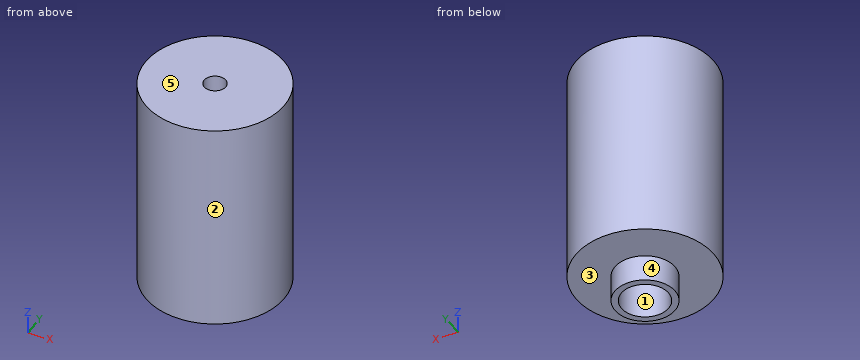
from build123d import *

# Parameters (mm, degrees)
SKETCH001_R   = 4.4
SKETCH001_R_2 = 2
PAD_DEPTH     = 4


with BuildPart() as part:
    # Sketch → Revolution (revolve)
    with BuildSketch(Plane.XZ):
        Polygon((-4.4, 0), (-5.6, 0), (-5.6, 5), (-12.85, 5), (-12.85, 45), (-4.4, 45), align=None)
    revolve(axis=Axis((0, 0, 0), (0, 0, 1)))

    # Sketch001 (on Face5 of Revolution) → Pad (new body)
    with BuildSketch(Plane(origin=(0, 0, 45), x_dir=(-1, 0, 0), z_dir=(0, 0, 1))):
        Circle(SKETCH001_R)
        Circle(SKETCH001_R_2, mode=Mode.SUBTRACT)
    extrude(amount=-PAD_DEPTH)


solid = part.part
Could you check a few things on this model? Use its own coordinates, in mm. Face numbers are marked on the shaded views. A direction names the side the tool comes from. Round coordinates to 2 decimals unless told otherwise and drop trailing zeros. Write each loop counter-clockwise with the first axis right and the second up, starting at its lowest first coordinate (ties: lowest second). Pieces come first, ordered by that corner, then holes. Notation, with made-up numbers: (4, 33) - (50, 33) arc R16 cw to (50, 50) - close; hole circle Ø3 at (22, -29.75). An arc over 180 degrees is marked (long way). Use a Markdown table: item, result.
Q1. Please list where these lines run through material, in increasing order: L1, parallel to Y at x = 0, z = 43.8; L2, parallel to Y at x = 0, z = 23.
Output values:
| item | result |
|---|---|
| L1 | -12.85 to -2, 2 to 12.85 |
| L2 | -12.85 to -4.4, 4.4 to 12.85 |
Q2. Thinking about a two-plate mould opening in Y: for the marked faces 1, 2 and 3, which applies, released by +Y, released by -Y, zero draft, split by the parting line, or undercut?
Output values:
| item | result |
|---|---|
| face 1 | undercut |
| face 2 | split by the parting line |
| face 3 | zero draft |
Q3. I want a section at A-A (y = 0). List the corners of the cut face in (x, z) for me, plus the area to 3 significant figures.
Output values:
| item | result |
|---|---|
| outline | (-12.85, 5) - (-5.6, 5) - (-5.6, 0) - (-4.4, 0) - (-4.4, 41) - (-2, 41) - (-2, 45) - (-12.85, 45) - close; (2, 41) - (4.4, 41) - (4.4, 0) - (5.6, 0) - (5.6, 5) - (12.85, 5) - (12.85, 45) - (2, 45) - close |
| area | 707 mm2 |
Q4. For the marked faces 4 and 5, which set-ups out of +Z, -Z, +X, -X, +Y, -Y let a thin tool reach every point of the face, with its end or its side?
Output values:
| item | result |
|---|---|
| face 4 | -Z |
| face 5 | +Z, +X, -X, +Y, -Y |
Q5. I want a section at D-D (x = -3.5). List the corners of the cut face in (y, z) for me, plus the area to 3 significant figures.
Output values:
| item | result |
|---|---|
| outline | (-12.36, 5) - (-4.37, 5) - (-4.37, 0) - (-2.67, 0) - (-2.67, 41) - (2.67, 41) - (2.67, 0) - (4.37, 0) - (4.37, 5) - (12.36, 5) - (12.36, 45) - (-12.36, 45) - close |
| area | 814 mm2 |
Q6. For pin 1 (1.5 mm diameter, centred on x = -6, y = 8.5, fed in from -Z); pin 2 (2 mm diameter, centred on x = -2, z = 7.5, fed in from -Y); pin 3 (10 mm diameter, centred on y = 6, z = 7.5, fed in from -X), each with a flat end and sliding along its axis, tell me the tip position at first contact or that it passes through.
Output values:
| item | result |
|---|---|
| pin 1 | z = 5 |
| pin 2 | y = -12.81 |
| pin 3 | x = -12.81 |
Q7. I want a section at C-C (z = 32). List the corners of the cut face in (x, y) for me, plus the area to 3 significant figures.
Output values:
| item | result |
|---|---|
| outline | circle Ø25.7 at (0, 0); hole circle Ø8.8 at (0, 0) |
| area | 458 mm2 |
